Here's how the part is built. I have some questions about the finished solid (model axes, mm). A direction names the side the tool comes from. Round coordinates to 2 decimals unless told otherwise and drop trailing zeros. Write each loop counter-clockwise with the first axis right and the second up, starting at its lowest first coordinate (ties: lowest second). Pieces come first, ordered by that corner, then holes. Notation, with made-up numbers: M -5.75,53.5 L 53.25,53.5 A13 cw 53.25,75.5 Z; hole C 66.25,11 d4. An arc over 180 degrees is marked long. Use one line per item in the form item = value. Start each with the question number.
Q1. I want a section at A-A on y = 22. List the corners of the cut face in (x, z) for me, and give its area (3 significant figures).
Q2. For faces 5 (the face through (7, 26.2, 32)), 6 (the face through (35.418, 7.205, 31.087)), which set-ups out of +Z, -Z, +X, -X, +Y, -Y let a thin tool reach every point of the face, with its end or its side?
Q3. I want a section at B-B on x = 35. List the corners of the cut face in (y, z) for me, and give its area (3 significant figures).
Q4. I'm going to push a flat-ended pin straight in: pin 1 Ø2 at (x, z) = (52, 13) entering from -Y. Where does the tip first touch, or does it pass through?
Q5. I want a section at C-C on z = 37. List the corners of the cut face in (x, y) for me.
Q6. I want a section at D-D on x = 42. List the corners of the cut face in (y, z) for me.
Q7. I need wall thicknesses on line 1 along X through (y, z) = (17.75, 44.5); line 2 along X through (y, z) = (9.5, 44.5); line 3 along Y through (x, z) = (17.5, 47). Which ranges of each line are inside material? Lowest first, please. Write a range as from..to.
Q8. We'd pull the mould along X, two halves only. Please class faces 1 (the face through (63, 26.2, 32)), 2 (the face through (35.374, 9.204, 1.014)), 3 (the face through (0, 13, 31)), 4 (the face through (70, 13, 31)): +X half, -X half, draft (parallel to the pull), parting line (faces both ways), or undercut.
```python
from build123d import *

# Parameters (mm, degrees)
BOSS_EXTRUDE1_DEPTH = 63
BOSS_EXTRUDE2_START = -2
BOSS_EXTRUDE2_DEPTH = 2


with BuildPart() as part:
    # Sketch1 → Boss-Extrude1 (new body)
    with BuildSketch(Plane.XY):
        with BuildLine():
            Line((0, 0), (70, 0))
            Line((70, 0), (70, 26.2))
            Line((70, 26.2), (54, 26.2))
            ThreePointArc((54, 26.2), (35, 7.2), (16, 26.2))
            Line((16, 26.2), (0, 26.2))
            Line((0, 26.2), (0, 0))
        make_face()
    extrude(amount=BOSS_EXTRUDE1_DEPTH)

    # Sketch2 → Boss-Extrude2 (add)
    with BuildSketch(Plane.XY.offset(63).offset(BOSS_EXTRUDE2_START)):
        with BuildLine():
            Line((18, 26.2), (16, 26.2))
            ThreePointArc((16, 26.2), (35, 7.2), (54, 26.2))
            Line((54, 26.2), (52, 26.2))
            ThreePointArc((52, 26.2), (35, 9.2), (18, 26.2))
        make_face()
    boss_extrude2 = extrude(amount=BOSS_EXTRUDE2_DEPTH)

    # Mirror1: Boss-Extrude2 across plane
    add(boss_extrude2.mirror(Plane(origin=(0, 0, 31.5), x_dir=(1, 0, 0), z_dir=(0, 0, -1))))


solid = part.part
```
Reported:
q1.outline = M 0,0 L 18.53,0 L 18.53,2 L 16.47,2 L 16.47,61 L 18.53,61 L 18.53,63 L 0,63 Z; M 51.47,0 L 70,0 L 70,63 L 51.47,63 L 51.47,61 L 53.53,61 L 53.53,2 L 51.47,2 Z
q1.area = 2,090 mm^2
q2.face_5 = +Z, -Z, +X, -X, +Y
q2.face_6 = +Y
q3.outline = M 0,0 L 9.2,0 L 9.2,2 L 7.2,2 L 7.2,61 L 9.2,61 L 9.2,63 L 0,63 Z
q3.area = 462 mm^2
q4.pin_1 = 0
q5.outline = M 0,0 L 70,0 L 70,26.2 L 54,26.2 A19 cw 16,26.2 L 0,26.2 Z
q6.outline = M 0,0 L 10.71,0 L 10.71,2 L 8.54,2 L 8.54,61 L 10.71,61 L 10.71,63 L 0,63 Z
q7.line_1 = 0..17.98, 52.02..70
q7.line_2 = 0..25.94, 44.06..70
q7.line_3 = 0..18.8
q8.face_1 = draft
q8.face_2 = undercut
q8.face_3 = -X half
q8.face_4 = +X half
